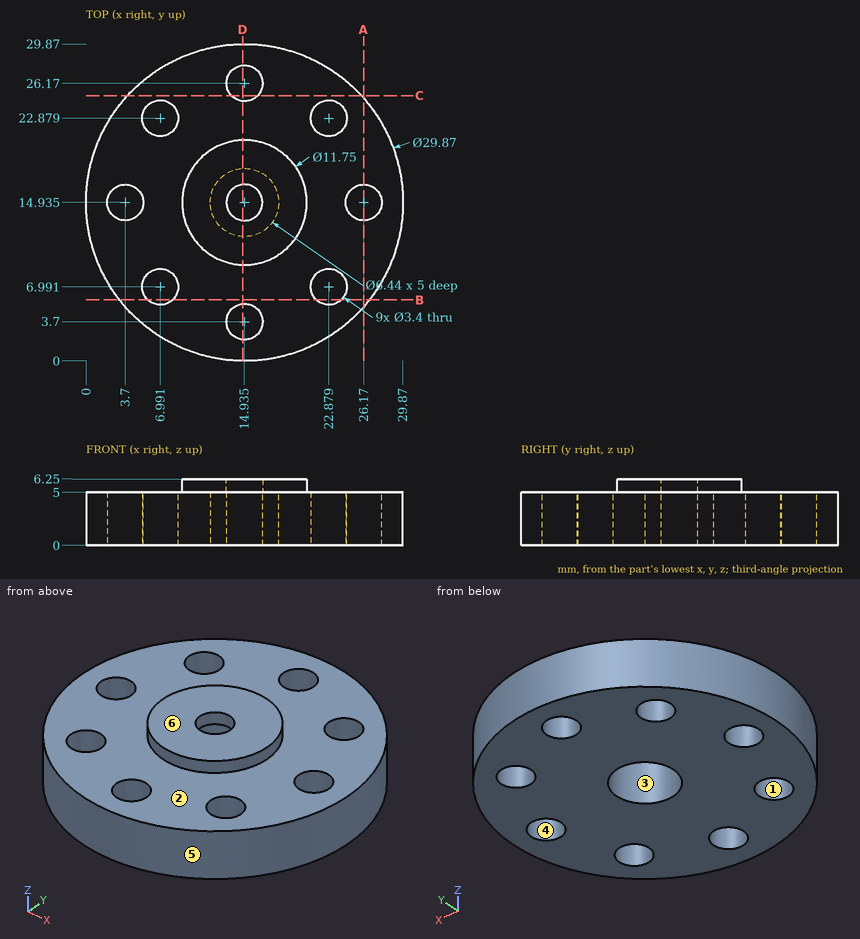
The drawing under review shows one solid part. Ordinate dimensions are in mm from its lowest x, y, z. A direction names the side the tool comes from. Round coordinates to 2 decimals unless told otherwise and drop trailing zeros. Order: outer loops, then holes, each group sorted by start corner. A loop starts at its lowest first (then second) coordinate and runs counter-clockwise, first axis right, second up. Notation, with made-up numbers: M -33.5,14 L -11.5,14 A19 cw -11.5,46 Z; hole C -10.5,30.5 d2. An arc over 180 degrees is marked long. Answer as CSV lines item,"result". Start each with the question number.
1) Add section D-D (x = 14.75). Give the number of separate pieces and of enclosed holes in the cut face.
2) The part is to be moulded in two halves that separate along X. For the marked faces 4, 5 and 6, say which applies: +X half, -X half, draft (parallel to the pull), parting line (faces both ways), or undercut.
3) Wall thickness on line 1 along Y through (x, z) = (24, 3) (1 decimal); line 2 along Y through (x, z) = (15.75, 4.75); line 3 along Y through (x, z) = (7, 4.5): over which ranges is each line inside the solid? List them lowest first. Write a range as [from, to].
4) Add section C-C (y = 25). Give the boundary of the cut face in (x, z), then the cut area to 3 significant figures.
5) Add section B-B (y = 5.75). Give the boundary of the cut face in (x, z).
6) Add section A-A (x = 26.17). Give the boundary of the cut face in (y, z) (1 decimal), then the cut area to 3 significant figures.
7) Tool access review of the marked faces 1, 2 and 3: name each direction out of +Z, -Z, +X, -X, +Y, -Y from which nothing blocks a thin tool from reaching the whole face with its end or side.
8) For pin 1 Ø3 at (x, y) = (14.935, 3.7) entering from -Z; pin 2 Ø2 at (x, z) = (22.5, 4) entering from -Y; pin 3 Ø6 at (x, y) = (6.5, 6) entering from +Z; pin 4 Ø2 at (x, z) = (11, 5) entering from -Y, all flat-tipped, find the tip position at first contact; note any pin that passes through.
Resolved:
1,separate pieces,"4"
1,enclosed holes,"0"
2,face 4,"undercut"
2,face 5,"parting line"
2,face 6,"draft"
3,line 1,"[3.1, 5.7], [8.3, 21.6], [24.2, 26.8]"
3,line 2,"[0.02, 2.21], [5.19, 11.82], [18.05, 24.68], [27.66, 29.85]"
3,line 3,"[2.28, 5.29], [8.69, 21.18], [24.58, 27.59]"
4,outline,"M 3.9,0 L 13.7,0 L 13.7,5 L 3.9,5 Z; M 16.17,0 L 25.97,0 L 25.97,5 L 16.17,5 Z"
4,area,"98.0 mm^2"
5,outline,"M 3.16,0 L 5.83,0 L 5.83,5 L 3.16,5 Z; M 8.15,0 L 21.72,0 L 21.72,5 L 8.15,5 Z; M 24.04,0 L 26.71,0 L 26.71,5 L 24.04,5 Z"
6,outline,"M 5.1,0 L 13.2,0 L 13.2,5 L 5.1,5 Z; M 16.6,0 L 24.8,0 L 24.8,5 L 16.6,5 Z"
6,area,"81.4 mm^2"
7,face 1,"+Z, -Z"
7,face 2,"+Z"
7,face 3,"-Z"
8,pin 1,"through"
8,pin 2,"y = 1.52"
8,pin 3,"z = 5"
8,pin 4,"y = 0.29"
